Geometry: final body of the model. Coordinates: model frame, mm. Give positions to 0.01 mm unless a question says otherwise; leave off trailing zeros. Loops run counter-clockwise (first coordinate to the right, second up) from the corner with the lowest first, then second, coordinate; pieces in that order, holes last. Notation, with made-up numbers: M -4,34 L 53,34 A32 ccw 53,66 Z; hole C -21.75,18.5 d2. An arc over 180 degrees is marked long. Put each result on its own line as item: value.
```python
from build123d import *

# Parameters (mm, degrees)
F0_W     = 235
F0_H     = 330
F0_W_2   = 40
F0_H_2   = 16
F0_W_3   = 18
F0_H_3   = 18
F1_DEPTH = 18
F2_SIZE  = 59
F3_R     = 10


with BuildPart() as f1:
    # F0 (on Front) → F1 (new body)
    with BuildSketch(Plane.XZ):
        Rectangle(F0_W, F0_H)
        with Locations((-87.5, -87)):
            Rectangle(F0_W_2, F0_H_2, mode=Mode.SUBTRACT)
        with Locations((-49, -136)):
            Rectangle(F0_W_3, F0_H_3, mode=Mode.SUBTRACT)
        with Locations((49, -136)):
            Rectangle(F0_W_3, F0_H_3, mode=Mode.SUBTRACT)
        with Locations((87.5, -87)):
            Rectangle(F0_W_2, F0_H_2, mode=Mode.SUBTRACT)
        with Locations((-49, 4)):
            Rectangle(F0_W_3, F0_H_3, mode=Mode.SUBTRACT)
        with Locations((-87.5, 147)):
            Rectangle(F0_W_2, F0_H_2, mode=Mode.SUBTRACT)
        with Locations((-49, 144)):
            Rectangle(F0_W_3, F0_H_3, mode=Mode.SUBTRACT)
        with Locations((49, 4)):
            Rectangle(F0_W_3, F0_H_3, mode=Mode.SUBTRACT)
        with Locations((49, 144)):
            Rectangle(F0_W_3, F0_H_3, mode=Mode.SUBTRACT)
        with Locations((87.5, 147)):
            Rectangle(F0_W_2, F0_H_2, mode=Mode.SUBTRACT)
    extrude(amount=F1_DEPTH)

    # F2
    f2_edges = [f1.edges().sort_by_distance(p)[0] for p in [
        (117.5, -9, -165),
        (-117.5, -9, -165),
    ]]
    chamfer(f2_edges, length=F2_SIZE)

    # F3
    f3_edges = [f1.edges().sort_by_distance(p)[0] for p in [
        (117.5, -9, 165),
        (117.5, -9, -106),
        (-117.5, -9, 165),
        (-117.5, -9, -106),
    ]]
    fillet(f3_edges, radius=F3_R)


solid = f1.part
```
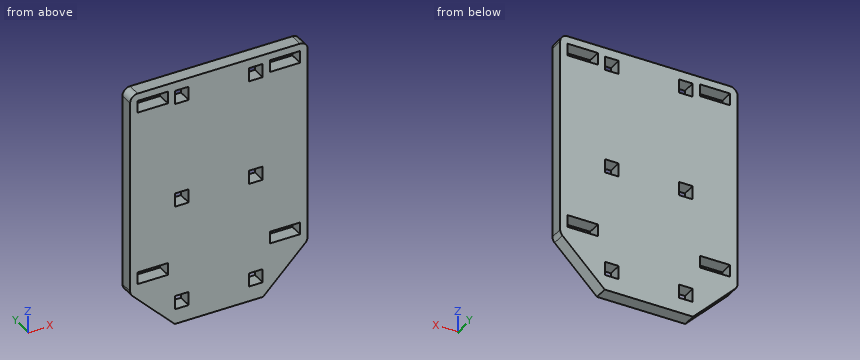
Item 1: Section B-B on x = -98. Output: boundary loops of the cut face in (y, z), then the cut area to 3 significant figures.
Output values:
outline: M -18,-125.5 L 0,-125.5 L 0,-95 L -18,-95 Z; M -18,-79 L 0,-79 L 0,139 L -18,139 Z; M -18,155 L 0,155 L 0,165 L -18,165 Z
area: 4,650 mm²
Item 2: Section C-C on y = -7.5. Count the separate pieces of the cut face and the enclosed holes in it, then the cut area to 3 significant figures.
Output values:
separate pieces: 1
enclosed holes: 10
area: 69,500 mm²
Item 3: Line query: probe 1 along X at (y, z) = (-2.25, -0.5); probe 2 along Z at (x, y) = (52, -4.5); probe 3 along Z at (x, y) = (-70, -11.5). Output: solid intervals per line, ascending. Write a range as [from, to].
Output values:
probe 1: [-117.5, -58], [-40, 40], [58, 117.5]
probe 2: [-165, -145], [-127, -5], [13, 135], [153, 165]
probe 3: [-153.5, -95], [-79, 139], [155, 165]
Item 4: Section A-A on x = 89.5. Output: boundary loops of the cut face in (y, z), then the cut area to 3 significant figures.
Output values:
outline: M -18,-134 L 0,-134 L 0,-95 L -18,-95 Z; M -18,-79 L 0,-79 L 0,139 L -18,139 Z; M -18,155 L 0,155 L 0,165 L -18,165 Z
area: 4,810 mm²
Item 5: Section D-D on x = 63.5. Output: boundary loops of the cut face in (y, z), then the cut area to 3 significant figures.
Output values:
outline: M -18,-160 L 0,-160 L 0,165 L -18,165 Z
area: 5,850 mm²
